Source: three-view drawing plus pictorial views. Frame: mm from the lowest corner of the part. A direction names the side the tool comes from. Round coordinates to 2 decimals unless told otherwise and drop trailing zeros. Loops run counter-clockwise (first coordinate to the right, second up) from the corner with the lowest first, then second, coordinate; pieces in that order, holes last. Notation, with made-up numbers: (-23.75, 2) -> (-3.75, 2) arc R5 cw to (-3.75, 8) -> close; hole circle Ø5 at (-24.5, 20). An arc over 180 degrees is marked (long way). Answer in a Markdown table with one row per item.
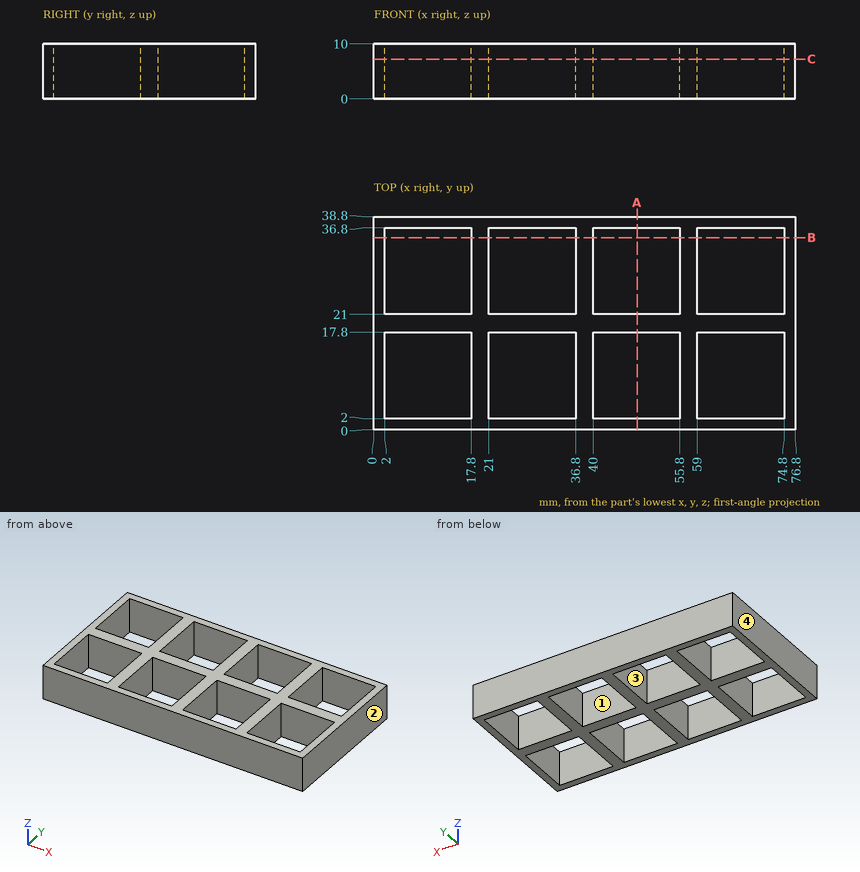
Item 1: Cut plane B-B (y = 35). Output: boundary loops of the cut face in (x, z), then the cut area to 3 significant figures.
Answer:
| item | result |
|---|---|
| outline | (0, 0) -> (2, 0) -> (2, 10) -> (0, 10) -> close; (17.8, 0) -> (21, 0) -> (21, 10) -> (17.8, 10) -> close; (36.8, 0) -> (40, 0) -> (40, 10) -> (36.8, 10) -> close; (55.8, 0) -> (59, 0) -> (59, 10) -> (55.8, 10) -> close; (74.8, 0) -> (76.8, 0) -> (76.8, 10) -> (74.8, 10) -> close |
| area | 136 mm² |
Item 2: Cut plane C-C (z = 7.25). Count the separate pieces of the cut face and the enclosed holes in it, then the cut area to 3 significant figures.
Answer:
| item | result |
|---|---|
| separate pieces | 1 |
| enclosed holes | 8 |
| area | 983 mm² |
Item 3: Cut plane A-A (x = 48). Output: boundary loops of the cut face in (y, z), then the cut area to 3 significant figures.
Answer:
| item | result |
|---|---|
| outline | (0, 0) -> (2, 0) -> (2, 10) -> (0, 10) -> close; (17.8, 0) -> (21, 0) -> (21, 10) -> (17.8, 10) -> close; (36.8, 0) -> (38.8, 0) -> (38.8, 10) -> (36.8, 10) -> close |
| area | 72.0 mm² |
Item 4: Line query: probe 1 along X at (y, z) = (36.5, 3.5); probe 2 along Y at (x, z) = (45, 1.25). Output: solid intervals per line, ascending. Write a range as [from, to].
Answer:
| item | result |
|---|---|
| probe 1 | x = [0, 2], [17.8, 21], [36.8, 40], [55.8, 59], [74.8, 76.8] |
| probe 2 | y = [0, 2], [17.8, 21], [36.8, 38.8] |
Item 5: Draft query along Y for the marked faces 1 and 2. Return one class per face: pulls with the +Y half, pulls with the -Y half, needs draft (parallel to the pull), parting line crosses it, or undercut.
Answer:
| item | result |
|---|---|
| face 1 | undercut |
| face 2 | needs draft |
Item 6: Reachability of the marked faces 3 and 4 from +Z, -Z, +X, -X, +Y, -Y: full face, straight path, thin tool, end or side. Return the list, or none.
Answer:
| item | result |
|---|---|
| face 3 | +Z, -Z |
| face 4 | +Z, -Z, -X, +Y, -Y |
Item 7: Pin query (flat end, axial travel): pin 1 Ø2 at (x, y) = (15, 31.5) entering from +Z. Return the tip coordinate at first contact, or that it passes through.
Answer:
| item | result |
|---|---|
| pin 1 | passes through |
